from build123d import *

# Parameters (mm, degrees)
F0_W     = 36
F0_H     = 37
F0_R     = 15
F1_DEPTH = 14
F0_R_2   = 12.5
F2_DEPTH = 3
F3_R     = 2.5
F4_DEPTH = 8


with BuildPart() as f1:
    # F0 (on Front) → F1 (new body)
    with BuildSketch(Plane.XZ):
        with Locations((0, -0.5)):
            Rectangle(F0_W, F0_H)
        Circle(F0_R, mode=Mode.SUBTRACT)
    extrude(amount=F1_DEPTH)

    # F0 (on Front) → F2 (join)
    with BuildSketch(Plane.XZ):
        with Locations((0, -0.5)):
            Rectangle(F0_W, F0_H)
        Circle(F0_R, mode=Mode.SUBTRACT)
        Circle(F0_R)
        Circle(F0_R_2, mode=Mode.SUBTRACT)
    extrude(amount=-F2_DEPTH)

    # F3 (on face) → F4 (cut)
    with BuildSketch(Plane(origin=(0, 0, -19), x_dir=(1, 0, 0), z_dir=(0, 0, -1))):
        with Locations((-13, 5.5)):
            Circle(F3_R)
        with Locations((13, 5.5)):
            Circle(F3_R)
    extrude(amount=-F4_DEPTH, mode=Mode.SUBTRACT)


solid = f1.part
Could you check a few things on this model? Use its own coordinates, in mm. A direction names the side the tool comes from. Coordinates: 2 decimals unless noted, no trailing zeros. Loops run counter-clockwise (first coordinate to the right, second up) from the corner with the lowest first, then second, coordinate; pieces in that order, holes last.
1. We'd pull the mould along Z, two halves only. Please class faces 4 (the face through (-13, -6, -11)), 5 (the face through (0, 3, -13)), 6 (the face through (-3.4, 0, 12.3)): released by +Z, released by -Z, zero draft, split by the parting line, or undercut.
2. For P1, Ø2.5, axis at x = -14, y = -5, coming from the -Z side, with a flat end and sliding along its axis, tell me the tip position at first contact or that it passes through.
3. I need wall thicknesses on L1, parallel to X at y = -5.5, z = -16.5; L2, parallel to Y at x = 13, z = -16.75; L3, parallel to X at y = -7, z = -16. Which ranges of each line are inside material? Lowest first, please.
4. For faces 1 (the face through (-18, -6, -1)), 2 (the face through (10.5, -5.6, -15.1)), 3 (the face through (-14.985, -6.902, 0.66)), which set-ups out of +Z, -Z, +X, -X, +Y, -Y let a thin tool reach every point of the face, with its end or its side?
5. Imagine slicing it at C-C (x = 11.5). Please give me the cut outline in (y, z), and give its area (3 significant figures).
6. Imagine slicing it at D-D (z = -14). Please give me the cut outline in (x, y), and give its area (3 significant figures).
7. Imagine slicing it at B-B (z = 0). Please give me the cut outline in (x, y).
8. Imagine slicing it at A-A (y = -5.5). Please give me the cut outline in (x, z), and give its area (3 significant figures).
Computed values:
1. face 4: released by -Z
1. face 5: zero draft
1. face 6: undercut
2. P1: stops at z = -11
3. L1: x = -18 to -15.5, -10.5 to 10.5, 15.5 to 18
3. L2: y = -14 to -8, -3 to 3
3. L3: x = -18 to -15, -11 to 11, 15 to 18
4. face 1: +Z, -Z, -X, +Y, -Y
4. face 2: -Z
4. face 3: -Y
5. outline: (-14, -19) - (-7.5, -19) - (-7.5, -11) - (-3.5, -11) - (-3.5, -19) - (3, -19) - (3, -4.9) - (0, -4.9) - (0, -9.63) - (-14, -9.63) - close; (-14, 9.63) - (0, 9.63) - (0, 4.9) - (3, 4.9) - (3, 18) - (-14, 18) - close
5. area: 298 mm2
6. outline: (-18, -14) - (-5.39, -14) - (-5.39, 0) - (5.39, 0) - (5.39, -14) - (18, -14) - (18, 3) - (-18, 3) - close; hole circle Ø5 at (-13, -5.5); hole circle Ø5 at (13, -5.5)
6. area: 422 mm2
7. outline: (-18, -14) - (-15, -14) - (-15, 0) - (-12.5, 0) - (-12.5, 3) - (-18, 3) - close; (12.5, 0) - (15, 0) - (15, -14) - (18, -14) - (18, 3) - (12.5, 3) - close
8. outline: (-18, -19) - (-15.5, -19) - (-15.5, -11) - (-10.5, -11) - (-10.5, -19) - (10.5, -19) - (10.5, -11) - (15.5, -11) - (15.5, -19) - (18, -19) - (18, 18) - (-18, 18) - close; hole circle Ø30 at (0, 0)
8. area: 545 mm2
